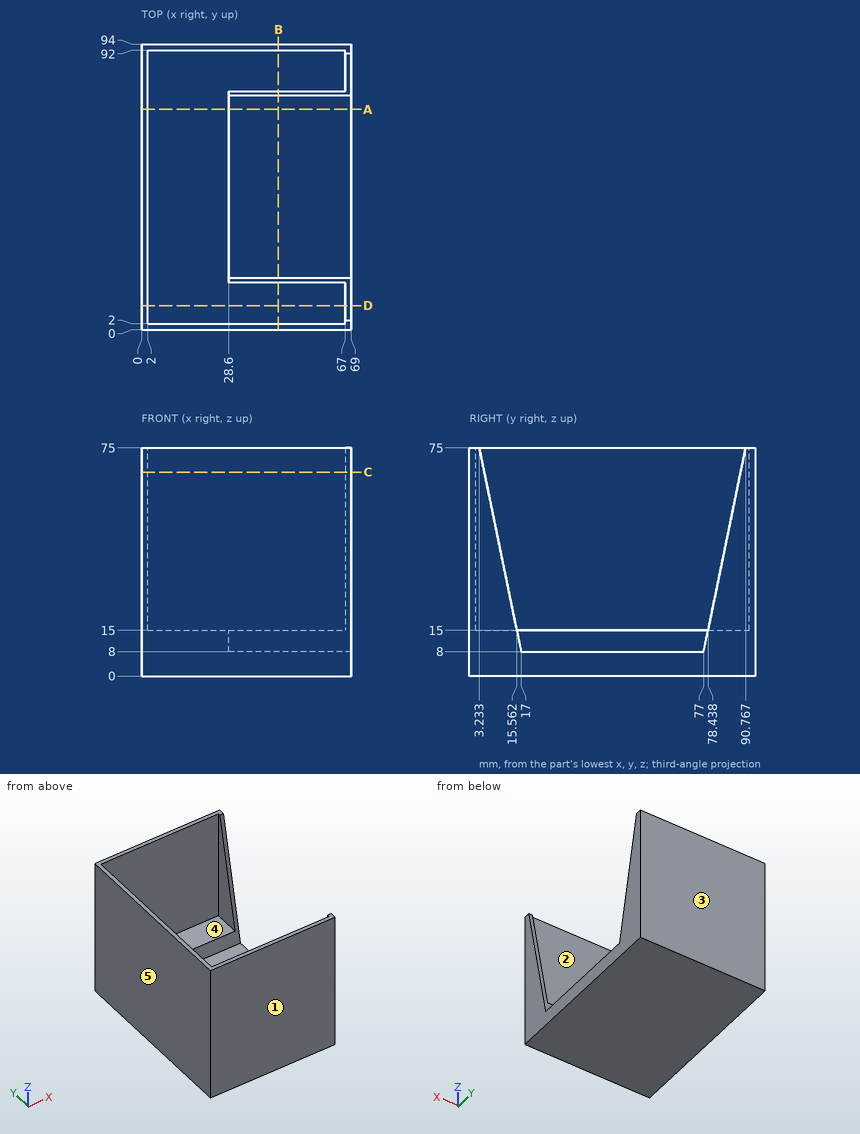
Geometry: see drawing. Coordinates: mm, zero at the bounding-box minimum. A direction names the side the tool comes from. Coordinates: 2 decimals unless noted, no trailing zeros. Order: outer loops, then holes, each group sorted by start corner. A loop starts at its lowest first (then second) coordinate and runs counter-clockwise, first axis right, second up. Notation, with made-up numbers: M 15,29.5 L 42,29.5 A10 ccw 42,40.5 Z; hole C 15.5,55 d9. An arc over 180 degrees is marked long. Write item = value, one per line. Start each with the question number.
(1) First-contact query: P1, Ø1.5, axis at y = 35, z = 63.5, coming from the +X side; P2, Ø2, axis at y = 44.5, z = 13, coming from the +X side. Flat tips, straight axial feed; report the tip coordinate or a pass-through.
(2) Section D-D on y = 8. Output: boundary loops of the cut face in (x, z), and give its area (3 significant figures).
(3) Pull-direction query (Y, two-part tool) for the marked faces 3, 4 and 5; classes: released by +Y, released by -Y, zero draft, split by the parting line, or undercut.
(4) Section C-C on z = 67. Output: boundary loops of the cut face in (x, y).
(5) Reachability of the marked faces 1 and 2 from +Z, -Z, +X, -X, +Y, -Y: full face, straight path, thin tool, end or side. Return the list, or none.
(6) Line query: line 1 along Y through (x, z) = (29.5, 58.5); line 2 along X through (y, z) = (87, 65); line 3 along Z through (x, y) = (38.5, 59). Output: solid intervals per line, ascending. Write a range as [from, to].
(7) Section B-B on x = 45. Output: boundary loops of the cut face in (y, z).
(8) Section A-A on y = 72.5. Output: boundary loops of the cut face in (x, z), and give its area (3 significant figures).
Result set:
q1.P1 = 2
q1.P2 = 28.6
q2.outline = M 0,0 L 69,0 L 69,51.8 L 67,51.8 L 67,15 L 2,15 L 2,75 L 0,75 Z
q2.area = 1,230 mm²
q3.face_3 = released by +Y
q3.face_4 = undercut
q3.face_5 = zero draft
q4.outline = M 0,0 L 69,0 L 69,4.88 L 67,4.88 L 67,2 L 2,2 L 2,92 L 67,92 L 67,89.12 L 69,89.12 L 69,94 L 0,94 Z
q5.face_1 = +Z, -Z, +X, -X, -Y
q5.face_2 = +Z
q6.line_1 = [0, 2], [92, 94]
q6.line_2 = [0, 2]
q6.line_3 = [0, 8]
q7.outline = M 0,0 L 94,0 L 94,75 L 92,75 L 92,15 L 78.44,15 L 77,8 L 17,8 L 15.56,15 L 2,15 L 2,75 L 0,75 Z
q8.outline = M 0,0 L 69,0 L 69,8 L 28.6,8 L 28.6,15 L 2,15 L 2,75 L 0,75 Z
q8.area = 872 mm²
